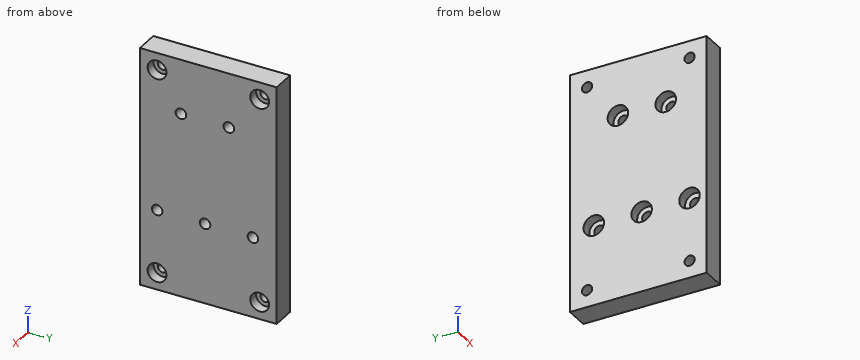
from build123d import *

# Parameters (mm, degrees)
SKETCH_1_W          = 70
SKETCH_1_H          = 40
EXTRUDE_3_DEPTH     = 6.9
SKETCH_2_R          = 1.5
CUT_EXTRUDE_1_DEPTH = 6.9
SKETCH_5_R          = 2.75
CUT_EXTRUDE_3_DEPTH = 3
SKETCH_6_R          = 1.52480842
SKETCH_6_R_2        = 1.55
CUT_EXTRUDE_4_DEPTH = 10
SKETCH_7_R          = 3
CUT_EXTRUDE_6_DEPTH = 3


with BuildPart() as part:
    # 草图1 → 凸台-拉伸3 (new body)
    with BuildSketch(Plane(origin=(0, 0, 0), x_dir=(0, 0, -1), z_dir=(1, 0, 0))):
        with Locations((35, 20)):
            Rectangle(SKETCH_1_W, SKETCH_1_H)
    extrude(amount=EXTRUDE_3_DEPTH)

    # 草图2 → 切除-拉伸1 (cut)
    with BuildSketch(Plane(origin=(6.9, 0, 0), x_dir=(0, 0, -1), z_dir=(1, 0, 0))):
        with BuildLine():
            ThreePointArc((6.5, 35), (6.060660172, 36.060660172), (5, 36.5))
            Line((5, 36.5), (5, 35))
            Line((5, 35), (3.5, 35))
            ThreePointArc((3.5, 35), (5, 33.5), (6.5, 35))
        make_face()
        with BuildLine():
            Line((5, 35), (5, 36.5))
            ThreePointArc((5, 36.5), (3.939339828, 36.060660172), (3.5, 35))
            Line((3.5, 35), (5, 35))
        make_face()
        with Locations((5, 5)):
            Circle(SKETCH_2_R)
        with Locations((65, 5)):
            Circle(SKETCH_2_R)
        with Locations((65, 35)):
            Circle(SKETCH_2_R)
    extrude(amount=-CUT_EXTRUDE_1_DEPTH, mode=Mode.SUBTRACT)

    # 草图5 → 切除-拉伸3 (cut)
    with BuildSketch(Plane(origin=(6.9, 0, 0), x_dir=(0, 0, -1), z_dir=(1, 0, 0))):
        with Locations((5, 35)):
            Circle(SKETCH_5_R)
        with Locations((5, 5)):
            Circle(SKETCH_5_R)
        with Locations((65, 35)):
            Circle(SKETCH_5_R)
        with Locations((65, 5)):
            Circle(SKETCH_5_R)
    extrude(amount=-CUT_EXTRUDE_3_DEPTH, mode=Mode.SUBTRACT)

    # 草图6 → 切除-拉伸4 (cut)
    with BuildSketch(Plane(origin=(6.9, 0, 0), x_dir=(0, 0, -1), z_dir=(1, 0, 0))):
        with Locations((46.461053437, 5.03563892)):
            Circle(SKETCH_6_R)
        with Locations((46.461053437, 19.03563892)):
            Circle(SKETCH_6_R_2)
        with Locations((46.461053437, 33.03563892)):
            Circle(SKETCH_6_R_2)
        with Locations((15.961053437, 25.98563892)):
            Circle(SKETCH_6_R_2)
        with Locations((15.961053437, 11.98563892)):
            Circle(SKETCH_6_R_2)
    extrude(amount=-CUT_EXTRUDE_4_DEPTH, mode=Mode.SUBTRACT)

    # 草图7 → 切除-拉伸6 (cut)
    with BuildSketch(Plane.ZY):
        with Locations((-46.461053437, 33.03563892)):
            Circle(SKETCH_7_R)
        with Locations((-46.461053437, 19.03563892)):
            Circle(SKETCH_7_R)
        with Locations((-46.461053437, 5.03563892)):
            Circle(SKETCH_7_R)
        with Locations((-15.961053437, 11.98563892)):
            Circle(SKETCH_7_R)
        with Locations((-15.961053437, 25.98563892)):
            Circle(SKETCH_7_R)
    extrude(amount=-CUT_EXTRUDE_6_DEPTH, mode=Mode.SUBTRACT)


solid = part.part
Can you work these out from the model? Positions are in its coordinate system, mm. Coordinates: 2 decimals unless noted, no trailing zeros. Write each loop counter-clockwise with the first axis right and the second up, starting at its lowest first coordinate (ties: lowest second). Pieces come first, ordered by that corner, then holes. Notation, with made-up numbers: (-19.5, -38.75) - (14.5, -38.75) arc R27 cw to (14.5, -10.75) - close; hole circle Ø8 at (-33, 24.25). An arc over 180 degrees is marked (long way). Return JSON: item names as keys, results as strings. Group by question number.
Item 1: If we section it at A-A (z = -65): Write out the boundary of the cut face in (x, y), then the cut area to 3 significant figures.
Item 2: If we section it at B-B (x = 6.25): Count the separate pieces of the cut face and the enclosed holes in it, then the cut area to 3 significant figures.
Item 3: Please list where these lines run through material, in increasing order: probe 1 along Y at (x, z) = (5.2, -65); probe 2 along Y at (x, z) = (2, -4); probe 3 along Z at (x, y) = (4.75, 6).
Item 4: I'm going to push flat-ended pins straight in: pin 1 Ø3 at (y, z) = (32, -47.5) entering from -X; pin 2 Ø2.5 at (y, z) = (5, -5) entering from +X; pin 3 Ø3 at (y, z) = (35.5, -6) entering from +X. Where does each tip first touch, or does it pass through?
Return value:
{
 "1": {"outline": "(0, 0) - (6.9, 0) - (6.9, 2.25) - (3.9, 2.25) - (3.9, 3.5) - (0, 3.5) - close; (0, 6.5) - (3.9, 6.5) - (3.9, 7.75) - (6.9, 7.75) - (6.9, 32.25) - (3.9, 32.25) - (3.9, 33.5) - (0, 33.5) - close; (0, 36.5) - (3.9, 36.5) - (3.9, 37.75) - (6.9, 37.75) - (6.9, 40) - (0, 40) - close", "area": "220 mm^2"},
 "2": {"separate pieces": "1", "enclosed holes": "9", "area": "2,670 mm^2"},
 "3": {"probe 1": "y = 0 to 2.25, 7.75 to 32.25, 37.75 to 40", "probe 2": "y = 0 to 3.88, 6.12 to 33.88, 36.12 to 40", "probe 3": "z = -70 to -67.56, -62.44 to -47.64, -45.28 to -7.56, -2.44 to 0"},
 "4": {"pin 1": "stops at x = 3", "pin 2": "passes through", "pin 3": "stops at x = 3.9"}
}
